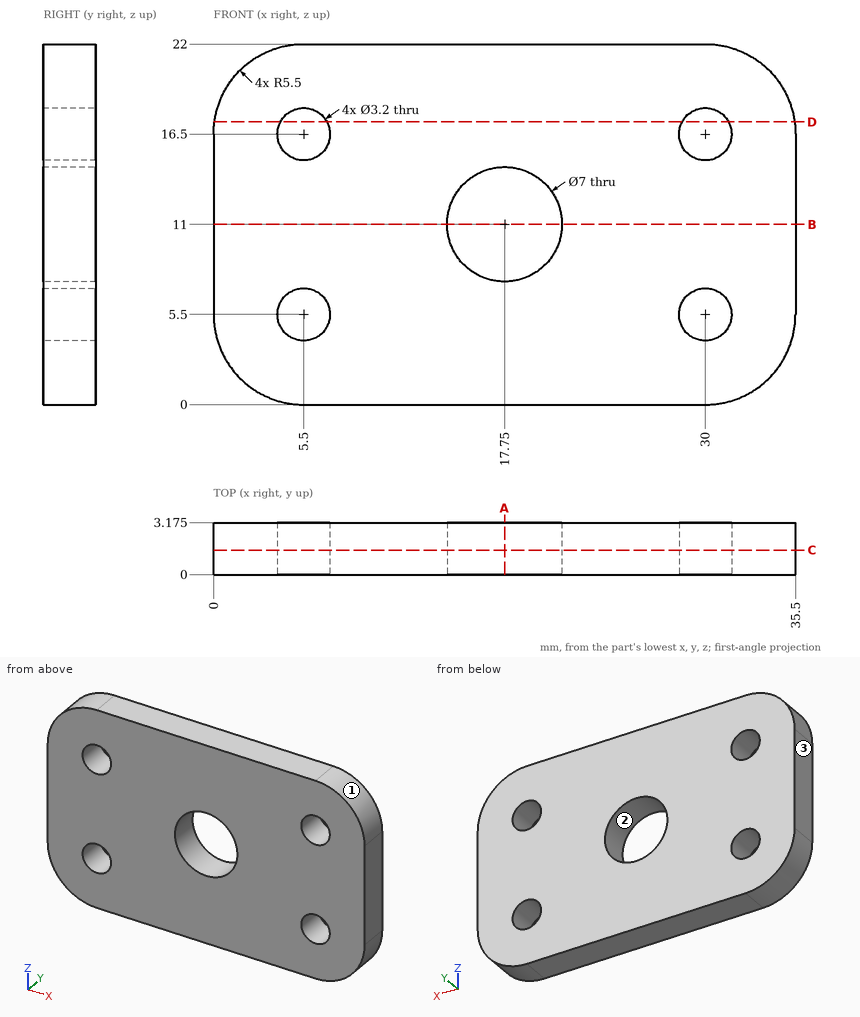
Geometry check sheet. Reference: drawing and pictorial views, mm from the part's lowest x, y, z. Give positions to 0.01 mm unless a question says otherwise; leave off trailing zeros. Order: outer loops, then holes, each group sorted by start corner. A loop starts at its lowest first (then second) coordinate and runs counter-clockwise, first axis right, second up. Notation, with made-up numbers: M 59.25,27 L 83.25,27 A24 cw 83.25,38 Z; hole C 7,70 d1. An arc over 180 degrees is marked long. Answer in a Markdown table with one row per item. Add a question column.
Q1. Sectioned sample at C-C, the plane y = 1.5. Record the boundary of the cut face in (x, z), and give its area (3 significant figures).
Q2. Sectioned sample at B-B, the plane z = 11. Record the boundary of the cut face in (x, y) (3 decimals), and give its area (3 significant figures).
Q3. Sectioned sample at D-D, the plane z = 17.25. Record the boundary of the cut face in (x, y) (3 decimals).
Q4. Sectioned sample at A-A, the plane x = 17.75. Record the boundary of the cut face in (y, z) (3 decimals).
Q5. Release check for a two-part mould opening along Z. For the marked faces 1, 2 and 3 record: released by +Z, released by -Z, zero draft, split by the parting line, or undercut.
Q6. Thickness scan on L1, parallel to X at y = 0.75, z = 5.5; L2, parallel to Z at x = 29, y = 1.25; L3, parallel to Z at x = 18, y = 2.05. Record the ranges inside material, lowest first.
Verdict:
| question | item | result |
|---|---|---|
| 1 | outline | M 0,5.5 A5.5 ccw 5.5,0 L 30,0 A5.5 ccw 35.5,5.5 L 35.5,16.5 A5.5 ccw 30,22 L 5.5,22 A5.5 ccw 0,16.5 Z; hole C 5.5,5.5 d3.2; hole C 5.5,16.5 d3.2; hole C 17.75,11 d7; hole C 30,5.5 d3.2; hole C 30,16.5 d3.2 |
| 1 | area | 684 mm² |
| 2 | outline | M 0,0 L 14.25,0 L 14.25,3.175 L 0,3.175 Z; M 21.25,0 L 35.5,0 L 35.5,3.175 L 21.25,3.175 Z |
| 2 | area | 90.5 mm² |
| 3 | outline | M 0.051,0 L 4.087,0 L 4.087,3.175 L 0.051,3.175 Z; M 6.913,0 L 28.587,0 L 28.587,3.175 L 6.913,3.175 Z; M 31.413,0 L 35.449,0 L 35.449,3.175 L 31.413,3.175 Z |
| 4 | outline | M 0,0 L 3.175,0 L 3.175,7.5 L 0,7.5 Z; M 0,14.5 L 3.175,14.5 L 3.175,22 L 0,22 Z |
| 5 | face 1 | released by +Z |
| 5 | face 2 | undercut |
| 5 | face 3 | zero draft |
| 6 | L1 | 0 to 3.9, 7.1 to 28.4, 31.6 to 35.5 |
| 6 | L2 | 0 to 4.25, 6.75 to 15.25, 17.75 to 22 |
| 6 | L3 | 0 to 7.51, 14.49 to 22 |
